The listing builds one solid part. Answer for the finished solid, in the listing's coordinates (mm). A direction names the side the tool comes from. Round coordinates to 2 decimals unless told otherwise and drop trailing zeros. Write each loop counter-clockwise with the first axis right and the second up, starting at its lowest first coordinate (ties: lowest second). Pieces come first, ordered by that corner, then holes. Notation, with made-up numbers: (39.5, 72.5) - (78.5, 72.5) arc R14 cw to (78.5, 88.5) - close; hole circle Ø5 at (0.5, 7.25). An arc over 180 degrees is marked (long way). Return JSON: item names as keys, results as strings. Group by question number.
(1) Find the intervals of material crossed by line 1 along X through (y, z) = (74, 2.05); line 2 along X through (y, z) = (143, 0.3); line 3 along Y through (x, z) = (86, 0.65), in increasing order. Write a range as [from, to].
(2) Which of the six approach directions +Z, -Z, +X, -X, +Y, -Y give full straight-line access (tool end or side, diameter ignored) to faces 1 (the flat face through (3, 12, 2)), 2 (the flat face through (31, 0, 1)), 3 (the flat face through (2, 50, 2))?
(3) Section C-C, the plane y = 22 is taken. Write down the section's boundary in (x, z), then the cut area to 3 significant figures.
(4) Determine the mould class of faces 4 (the flat face through (3.935, 112, 2)), 5 (the flat face through (44, 76, 3)), 6 (the flat face through (1, 25, 2)) for opening direction Y: +Y half, -Y half, draft (parallel to the pull), parting line (faces both ways), or undercut.
(5) Each of these flat-tipped pins is pushed along its axis until it touches: pin 1 (0.9 mm diameter, centred on y = 59.5, z = 1.5, fed in from -X); pin 2 (0.9 mm diameter, centred on y = 13.5, z = 2, fed in from -X). Where does it stop, or does it pass through?
(6) Section A-A, the plane z = 1.7 is taken. Write down the section's boundary in (x, y), then the cut area to 3 significant figures.
(7) Section B-B, the plane y = 102.5 is taken. Write down the section's boundary in (x, z).
```python
from build123d import *

# Parameters (mm, degrees)
ESQUISSE1_W             = 90
ESQUISSE1_H             = 150
BOSS_EXTRU_2_DEPTH      = 3
ESQUISSE3_W             = 3.935197626
ESQUISSE3_H             = 25
ESQUISSE3_W_2           = 3
ENL_V_MAT_EXTRU_1_DEPTH = 3
CONG_1_R                = 30


with BuildPart() as part:
    # Esquisse1 → Boss.-Extru.2 (new body)
    with BuildSketch(Plane.XY):
        with Locations((45, 75)):
            Rectangle(ESQUISSE1_W, ESQUISSE1_H)
    extrude(amount=BOSS_EXTRU_2_DEPTH)

    # Esquisse3 → Enlèv. mat.-Extru.1 (cut)
    with BuildSketch(Plane.XY.offset(3)):
        with Locations((1.967598813, 112.5)):
            Rectangle(ESQUISSE3_W, ESQUISSE3_H)
        with Locations((1.967598813, 62.5)):
            Rectangle(ESQUISSE3_W, ESQUISSE3_H)
        with Locations((1.5, 12.5)):
            Rectangle(ESQUISSE3_W_2, ESQUISSE3_H)
    extrude(amount=-ENL_V_MAT_EXTRU_1_DEPTH, mode=Mode.SUBTRACT)

    # Congé1
    cong_1_edges = [part.edges().sort_by_distance(p)[0] for p in [
        (90, 0, 1.5),
        (90, 150, 1.5),
    ]]
    fillet(cong_1_edges, radius=CONG_1_R)


solid = part.part
```
Working result:
{
 "1": {"line 1": "x = [3.94, 90]", "line 2": "x = [0, 79.26]", "line 3": "y = [15.03, 134.97]"},
 "2": {"face 1": "+Z, -Z, -X, -Y", "face 2": "+Z, -Z, +X, -X, -Y", "face 3": "+Z, -Z, -X"},
 "3": {"outline": "(3, 0) - (88.91, 0) - (88.91, 3) - (3, 3) - close", "area": "258 mm^2"},
 "4": {"face 4": "undercut", "face 5": "draft", "face 6": "-Y half"},
 "5": {"pin 1": "stops at x = 3.94", "pin 2": "stops at x = 3"},
 "6": {"outline": "(0, 25) - (3, 25) - (3, 0) - (60, 0) arc R30 ccw to (90, 30) - (90, 120) arc R30 ccw to (60, 150) - (0, 150) - (0, 125) - (3.94, 125) - (3.94, 100) - (0, 100) - (0, 75) - (3.94, 75) - (3.94, 50) - (0, 50) - close", "area": "12,800 mm^2"},
 "7": {"outline": "(3.94, 0) - (90, 0) - (90, 3) - (3.94, 3) - close"}
}
